Model file for the job. Use its own axes, mm. Face numbers are marked on the shaded views. A direction names the side the tool comes from. Give positions to 0.01 mm unless a question says otherwise; leave off trailing zeros. Loops run counter-clockwise (first coordinate to the right, second up) from the corner with the lowest first, then second, coordinate; pieces in that order, holes last. Notation, with made-up numbers: (51, 84.5) - (93, 84.5) arc R15 cw to (93, 107.5) - close; hole circle Ø7 at (-3.5, -11.75). An arc over 180 degrees is marked (long way). Answer as CSV lines item,"result". Start each with the question number.
Item 1: Pin check, flat tip, straight feed: pin 1 (2 mm diameter, centred on y = -26, z = 20.5, fed in from -X). Stop position of the tip, or through.
Item 2: Saw through at C-C on z = 0. State how many separate pieces and enclosed holes the cut face has, plus the area to 3 significant figures.
Item 3: Pull direction Y, two halves, no side cores. Call the marked faces 3, 4 and 5: pulls with the +Y half, pulls with the -Y half, needs draft (parallel to the pull), parting line crosses it, or undercut.
Item 4: Saw through at B-B on y = 0. Give the cut face in (x, z), plus the area to 3 significant figures.
Item 5: Drill centre lines: L1, parallel to Z at x = 23.2, y = 0; L2, parallel to Y at x = 23, z = 0; L3, parallel to X at y = -75.95, z = 0. Where is each one in solid material? Low to high. Write a range as from..to.
Item 6: Tool access for the marked faces 1 and 2: list every direction of +Z, -Z, +X, -X, +Y, -Y with a clear straight run to the whole face (end or side of a thin tool).
Item 7: Saw through at A-A on x = -36. Give the cut face in (y, z).
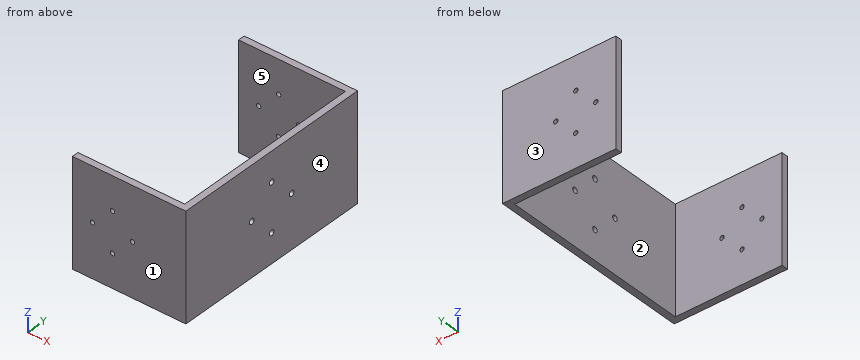
Autodesk Inventor part; units mm, degrees
ref_plane "YZ Plane" through (0, 0, 0) normal (1, 0, 0) x (0, 1, 0)
ref_plane "XZ Plane" through (0, 0, 0) normal (0, 1, 0) x (-1, 0, 0)
ref_plane "XY Plane" through (0, 0, 0) normal (0, 0, 1) x (1, 0, 0)
sketch "Sketch1" plane through (0, 0, 0) normal (0, 0, 1) x (1, 0, 0)
  line L0 (20.183, 72.5) -> (20.183, -72.5)
  line L1 (20.183, 72.5) -> (165.183, 72.5) construction
  line L2 (20.183, -72.5) -> (-59.817, -72.5)
  line L3 (-59.817, -72.5) -> (-59.817, -77.5)
  line L4 (-59.817, -72.5) -> (-54.817, -72.5) construction
  line L5 (-59.817, -77.5) -> (25.183, -77.5)
  line L6 (25.183, -77.5) -> (25.183, 77.5)
  line L7 (25.183, 77.5) -> (-59.817, 77.5)
  line L8 (-59.817, 77.5) -> (-59.817, 72.5)
  line L9 (-59.817, 72.5) -> (20.183, 72.5)
  point P0 (0, 0)
  dimension "d0" = 145
  dimension "d1" = 90
  dimension "d2" = 80
  dimension "d3" = 90
  dimension "d4" = 5
  dimension "d5" = 90
  dimension "d6" = 85
  dimension "d7" = 90
  dimension "d8" = 155
  dimension "d9" = 90
  dimension "d10" = 85
  dimension "d11" = 90
  dimension "d12" = 5
  dimension "d13" = 90
  dimension "d45" = 72.5
extrude "Extrusion1" add sketch "Sketch1" along normal mid plane 80
sketch "Sketch2" plane through (25.183, -77.5, 40) normal (1, 0, 0) x (0, 0, -1)
  line L0 (0, 0) -> (0, 155)
  line L1 (0, 150) -> (0, 5)
  line L2 (0, 77.5) -> (80, 77.5) construction
  line L3 (80, 5) -> (80, 150)
  line L4 (80, 0) -> (0, 0)
  line L5 (40, 37.5) -> (40, 117.5) construction
  line L6 (80, 77.5) -> (0, 77.5) construction
  line L7 (40, 117.5) -> (40, 37.5) construction
  point P0 (40, 77.5)
  point P1 (40, 95.534)
  point P2 (40, 77.5)
  point P3 (40, 77.5)
  point P4 (21.966, 77.5)
  point P5 (40, 77.5)
  point P6 (40, 59.466)
  point P7 (40, 77.5)
  point P8 (58.034, 77.5)
  dimension "d16" = 40
  dimension "d17" = 77.5
  dimension "d18" = 18.034
  dimension "d21" = 360
hole "Hole1" at (25.183, 18.034, 0) at (25.183, 0, 18.034) at (25.183, -18.034, 0) at (25.183, 0, -18.034) direction (-1, 0, 0) diameter 4.134 end through all
sketch "Sketch3" plane through (-59.817, 77.5, 40) normal (0, 1, 0) x (1, 0, 0)
  line L0 (60, 80) -> (0, 80)
  line L1 (30, 80) -> (30, 0) construction
  line L2 (60, 0) -> (0, 0)
  line L3 (30, 80) -> (120, 80) construction
  line L4 (85, 80) -> (85, 0)
  line L5 (85, 0) -> (0, 0)
  line L6 (0, 80) -> (85, 80)
  point P0 (59.817, 40)
  point P1 (15, 40)
  point P2 (30, 40)
  point P3 (30, 25)
  point P4 (45, 40)
  point P5 (30, 55)
  dimension "d30" = 90
  dimension "d31" = 55
  dimension "d32" = 40
  dimension "d33" = 15
  dimension "d36" = 360
hole "Hole2" at (-14.817, 77.5, 0) at (-29.817, 77.5, 15) at (-44.817, 77.5, 0) at (-29.817, 77.5, -15) direction (0, -1, 0) diameter 3.302 end through all
properties part number "sidebracket"
Responses:
1,pin 1,"x = 20.18"
2,separate pieces,"7"
2,enclosed holes,"0"
2,area,"1,470 mm2"
3,face 3,"pulls with the +Y half"
3,face 4,"needs draft"
3,face 5,"undercut"
4,outline,"(20.18, -40) - (25.18, -40) - (25.18, -20.1) - (20.18, -20.1) - close; (20.18, -15.97) - (25.18, -15.97) - (25.18, 15.97) - (20.18, 15.97) - close; (20.18, 20.1) - (25.18, 20.1) - (25.18, 40) - (20.18, 40) - close"
4,area,"359 mm2"
5,L1,"-40..-20.1, -15.97..15.97, 20.1..40"
5,L2,"-77.5..-20.1, -15.97..15.97, 20.1..77.5"
5,L3,"-59.82..-46.47, -43.17..-16.47, -13.17..25.18"
6,face 1,"+Z, -Z, +X, -X, -Y"
6,face 2,"+Z, -Z, -X"
7,outline,"(-77.5, -40) - (-72.5, -40) - (-72.5, 40) - (-77.5, 40) - close; (72.5, -40) - (77.5, -40) - (77.5, 40) - (72.5, 40) - close"
